Source: CAD feature listing. Evaluate the final solid. Frame: model axes, mm. Give positions to 0.01 mm unless a question says otherwise; leave off trailing zeros. Loops run counter-clockwise (first coordinate to the right, second up) from the corner with the lowest first, then second, coordinate; pieces in that order, holes last. Notation, with made-up numbers: M 1,82.5 L 26,82.5 A19 cw 26,88.5 Z; hole C 29.25,38.25 d11. An arc over 180 degrees is marked long. Write item = value, one per line.
from build123d import *

# Parameters (mm, degrees)
SKETCH1_W                = 80
SKETCH1_H                = 80
BOSS_EXTRUDE1_DEPTH      = 3.175
CUT_EXTRUDE3_START       = -3.175
CUT_EXTRUDE3_OUTLINE_W   = 3.175
CUT_EXTRUDE3_OUTLINE_H   = 5.333333334
CUT_EXTRUDE3_OUTLINE_H_2 = 5.333333333
CUT_EXTRUDE3_OUTLINE_W_2 = 5.333333334
CUT_EXTRUDE3_OUTLINE_H_3 = 3.175
CUT_EXTRUDE3_OUTLINE_W_3 = 5.333333333
CUT_EXTRUDE3_DEPTH       = 3.175


# Read off the part's stored shape, not the designer's step: Cut-Extrude3
with BuildPart() as part:
    # Sketch1 → Boss-Extrude1 (new body)
    with BuildSketch(Plane(origin=(0, 0, 0), x_dir=(1, 0, 0), z_dir=(0, 1, 0))):
        Rectangle(SKETCH1_W, SKETCH1_H)
    extrude(amount=BOSS_EXTRUDE1_DEPTH)

    # Cut-Extrude3 outline → Cut-Extrude3 (cut)
    with BuildSketch(Plane(origin=(0, 3.175, 0), x_dir=(1, 0, 0), z_dir=(0, 1, 0)).offset(CUT_EXTRUDE3_START)):
        with Locations((-38.4125, 32)):
            Rectangle(CUT_EXTRUDE3_OUTLINE_W, CUT_EXTRUDE3_OUTLINE_H)
        with Locations((-38.4125, 21.333333334)):
            Rectangle(CUT_EXTRUDE3_OUTLINE_W, CUT_EXTRUDE3_OUTLINE_H_2)
        with Locations((-32, 38.4125)):
            Rectangle(CUT_EXTRUDE3_OUTLINE_W_2, CUT_EXTRUDE3_OUTLINE_H_3)
        with Locations((-38.4125, 10.666666666)):
            Rectangle(CUT_EXTRUDE3_OUTLINE_W, CUT_EXTRUDE3_OUTLINE_H_2)
        with Locations((-21.333333334, 38.4125)):
            Rectangle(CUT_EXTRUDE3_OUTLINE_W_3, CUT_EXTRUDE3_OUTLINE_H_3)
        with Locations((-38.4125, 0)):
            Rectangle(CUT_EXTRUDE3_OUTLINE_W, CUT_EXTRUDE3_OUTLINE_H)
        with Locations((-10.666666666, 38.4125)):
            Rectangle(CUT_EXTRUDE3_OUTLINE_W_3, CUT_EXTRUDE3_OUTLINE_H_3)
        with Locations((-38.4125, -10.666666666)):
            Rectangle(CUT_EXTRUDE3_OUTLINE_W, CUT_EXTRUDE3_OUTLINE_H_2)
        with Locations((0, 38.4125)):
            Rectangle(CUT_EXTRUDE3_OUTLINE_W_2, CUT_EXTRUDE3_OUTLINE_H_3)
        with Locations((-38.4125, -21.333333334)):
            Rectangle(CUT_EXTRUDE3_OUTLINE_W, CUT_EXTRUDE3_OUTLINE_H_2)
        with Locations((10.666666666, 38.4125)):
            Rectangle(CUT_EXTRUDE3_OUTLINE_W_3, CUT_EXTRUDE3_OUTLINE_H_3)
        with Locations((-38.4125, -32)):
            Rectangle(CUT_EXTRUDE3_OUTLINE_W, CUT_EXTRUDE3_OUTLINE_H)
        with Locations((21.333333334, 38.4125)):
            Rectangle(CUT_EXTRUDE3_OUTLINE_W_3, CUT_EXTRUDE3_OUTLINE_H_3)
        with Locations((32, 38.4125)):
            Rectangle(CUT_EXTRUDE3_OUTLINE_W_2, CUT_EXTRUDE3_OUTLINE_H_3)
        with Locations((-32, -38.4125)):
            Rectangle(CUT_EXTRUDE3_OUTLINE_W_2, CUT_EXTRUDE3_OUTLINE_H_3)
        with Locations((-21.333333334, -38.4125)):
            Rectangle(CUT_EXTRUDE3_OUTLINE_W_3, CUT_EXTRUDE3_OUTLINE_H_3)
        with Locations((38.4125, 32)):
            Rectangle(CUT_EXTRUDE3_OUTLINE_W, CUT_EXTRUDE3_OUTLINE_H)
        with Locations((-10.666666666, -38.4125)):
            Rectangle(CUT_EXTRUDE3_OUTLINE_W_3, CUT_EXTRUDE3_OUTLINE_H_3)
        with Locations((38.4125, 21.333333334)):
            Rectangle(CUT_EXTRUDE3_OUTLINE_W, CUT_EXTRUDE3_OUTLINE_H_2)
        with Locations((0, -38.4125)):
            Rectangle(CUT_EXTRUDE3_OUTLINE_W_2, CUT_EXTRUDE3_OUTLINE_H_3)
        with Locations((38.4125, 10.666666666)):
            Rectangle(CUT_EXTRUDE3_OUTLINE_W, CUT_EXTRUDE3_OUTLINE_H_2)
        with Locations((10.666666666, -38.4125)):
            Rectangle(CUT_EXTRUDE3_OUTLINE_W_3, CUT_EXTRUDE3_OUTLINE_H_3)
        with Locations((38.4125, 0)):
            Rectangle(CUT_EXTRUDE3_OUTLINE_W, CUT_EXTRUDE3_OUTLINE_H)
        with Locations((21.333333334, -38.4125)):
            Rectangle(CUT_EXTRUDE3_OUTLINE_W_3, CUT_EXTRUDE3_OUTLINE_H_3)
        with Locations((38.4125, -10.666666666)):
            Rectangle(CUT_EXTRUDE3_OUTLINE_W, CUT_EXTRUDE3_OUTLINE_H_2)
        with Locations((32, -38.4125)):
            Rectangle(CUT_EXTRUDE3_OUTLINE_W_2, CUT_EXTRUDE3_OUTLINE_H_3)
        with Locations((38.4125, -21.333333334)):
            Rectangle(CUT_EXTRUDE3_OUTLINE_W, CUT_EXTRUDE3_OUTLINE_H_2)
        with Locations((38.4125, -32)):
            Rectangle(CUT_EXTRUDE3_OUTLINE_W, CUT_EXTRUDE3_OUTLINE_H)
    extrude(amount=CUT_EXTRUDE3_DEPTH, mode=Mode.SUBTRACT)


solid = part.part
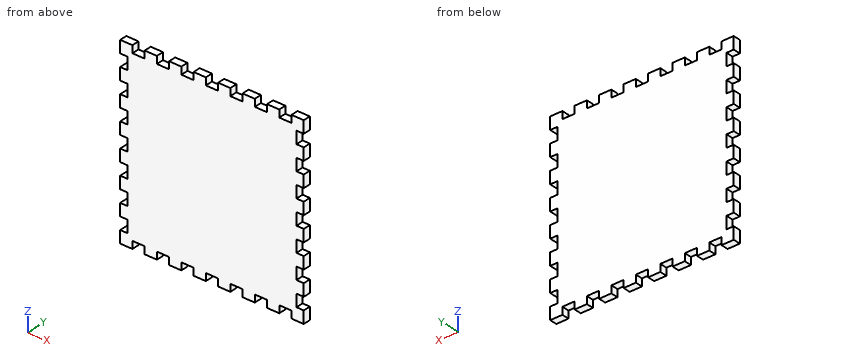
1. Cut plane B-B, the plane x = -20.5. Return the cut outline in (y, z) (3 decimals), then the cut area to 3 significant figures.
Derived:
outline = M 0,-36.825 L 3.175,-36.825 L 3.175,36.825 L 0,36.825 Z
area = 234 mm²
2. First-contact query: pin 1 Ø1 at (y, z) = (2, 22.5) entering from +X (3 decimals); pin 2 Ø1 at (x, y) = (10, 2) entering from +Z (3 decimals); pin 3 Ø1.6 at (y, z) = (1, 31.5) entering from -X (3 decimals). Flat tips, straight axial feed; report the tip coordinate or a pass-through.
Derived:
pin_1 = 36.825
pin_2 = 36.825
pin_3 = -36.825
3. Material intervals for probe 1 along Z at (x, y) = (-20.5, 2.7) (3 decimals), sorted ascending. Write a range as from..to.
Derived:
probe_1 = -36.825..36.825
4. Cut plane A-A, the plane z = 20.5. Return the cut outline in (x, y) (3 decimals), then the cut area to 3 significant figures.
Derived:
outline = M -36.825,0 L 36.825,0 L 36.825,3.175 L -36.825,3.175 Z
area = 234 mm²
